Read the model definition and answer for the solid it produces. Units are mm, in the model's axes. A direction names the side the tool comes from. Give positions to 0.01 mm unless a question says otherwise; leave off trailing zeros. Write each loop counter-clockwise with the first axis right and the second up, starting at its lowest first coordinate (ties: lowest second). Pieces come first, ordered by that corner, then holes.
```python
from build123d import *

# Parameters (mm, degrees)
F3_DEPTH = 38.1
F4_W     = 88.9
F4_H     = 88.9
F5_DEPTH = 19.05
F7_W     = 114.3
F7_H     = 254
F8_DEPTH = 38.1


with BuildPart() as f3:
    # F2 (on offset) → F3 (new body)
    with BuildSketch(Plane.YZ.offset(19.05)):
        Polygon((729.5686676615, 1263.65), (652.579009265, 1308.1), (-102.6528778619, 0), (-610.6528778619, 0), (-610.6528778619, -88.9), (729.5686676615, -88.9), (729.5686676615, 0), (602.5686676615, 0), (301.2843338307, 521.8397737194), align=None)
        Polygon((499.9157897996, 0), (0, 0), (249.9578948998, 432.9397737194), align=None, mode=Mode.SUBTRACT)
    extrude(amount=F3_DEPTH)

    # F4 (on Right) → F5 (join, through all)
    with BuildSketch(Plane.YZ):
        with Locations((685.1186676615, -44.45)):
            Rectangle(F4_W, F4_H)
        Polygon((-559.8528778619, 0), (-610.6528778619, 0), (-610.6528778619, -88.9), (-470.9528778619, -88.9), align=None)
        Polygon((0, -88.9), (0, 0), (-102.6528778619, 0), (-153.9793167929, -88.9), align=None)
    extrude(amount=F5_DEPTH)

    # F6: F3 across plane


with BuildPart() as f3_1:
    add(f3.part)
    add(f3.part.mirror(Plane.YZ))

    # F7 (on face) → F8 (join)
    with BuildSketch(Plane(origin=(0, 0, 0), x_dir=(-1, 0, 0), z_dir=(0, 0.8660254038, -0.5))):
        with Locations((0, 1332.1373353229)):
            Rectangle(F7_W, F7_H)
    extrude(amount=F8_DEPTH)


solid = f3_1.part
```
Item 1: Section C-C (z = 476.5) is taken. Write down the section's boundary in (x, y).
Result set:
outline: (-57.15, 172.45) - (-19.05, 172.45) - (-19.05, 327.46) - (-57.15, 327.46) - close; (19.05, 172.45) - (57.15, 172.45) - (57.15, 327.46) - (19.05, 327.46) - close
Item 2: Section D-D (y = 321) is taken. Write down the section's boundary in (x, z).
Result set:
outline: (-57.15, -88.9) - (-19.05, -88.9) - (-19.05, 0) - (-57.15, 0) - close; (-57.15, 309.89) - (-19.05, 309.89) - (-19.05, 487.69) - (-57.15, 487.69) - close; (-57.15, 555.99) - (-19.05, 555.99) - (-19.05, 733.79) - (-57.15, 733.79) - close; (19.05, -88.9) - (57.15, -88.9) - (57.15, 0) - (19.05, 0) - close; (19.05, 309.89) - (57.15, 309.89) - (57.15, 487.69) - (19.05, 487.69) - close; (19.05, 555.99) - (57.15, 555.99) - (57.15, 733.79) - (19.05, 733.79) - close
Item 3: Find the intervals of material crossed by line 1 along Z through (x, y) = (-42, 465.5); line 2 along Z through (x, y) = (-32.5, 199); line 3 along Z through (x, y) = (34.5, 283), in increasing order.
Result set:
line 1: z = -88.9 to 0, 59.61 to 237.41, 806.27 to 984.07
line 2: z = -88.9 to 0, 344.68 to 522.48
line 3: z = -88.9 to 0, 375.71 to 667.97
Item 4: Determine the mould class of faces 1 (the flat face through (-37.833, 373.187, 219.5)), 2 (the flat face through (-37.83, 280.25, 663.21)), 3 (the flat face through (-57.15, 294, 368)) for opening direction Z: pulls with the +Z half, pulls with the -Z half, needs draft (parallel to the pull), parting line crosses it, or undercut.
Result set:
face 1: undercut
face 2: pulls with the +Z half
face 3: needs draft
Item 5: Which of the six approach directions +Z, -Z, +X, -X, +Y, -Y give full straight-line access (tool end or side, diameter ignored) to faces 4 (the flat face through (19.05, -334, -44)), 5 (the flat face through (0, -51, 0)), 6 (the flat face through (0.267, 666.958, 1155.205)), 7 (the flat face through (0.8, 699.95, 1136.15)), 8 (the flat face through (38, 253, 0))?
Result set:
face 4: +Z
face 5: +Z, +Y, -Y
face 6: +Z, -Y
face 7: +X, -X, +Y
face 8: +X, -X
Item 6: Section B-B (x = -40.5) is taken. Write down the section's boundary in (y, z), and give its area (3 significant figures).
Result set:
outline: (-610.65, -88.9) - (729.57, -88.9) - (729.57, 0) - (602.57, 0) - (301.28, 521.84) - (602.57, 1043.68) - (635.56, 1024.63) - (762.56, 1244.6) - (652.58, 1308.1) - (-102.65, 0) - (-610.65, 0) - close; hole (0, 0) - (499.92, 0) - (249.96, 432.94) - close
area: 310,000 mm2
Item 7: Section A-A (y = -202.5) is taken. Write down the section's boundary in (x, z), and give its area (3 significant figures).
Result set:
outline: (-57.15, -88.9) - (-19.05, -88.9) - (-19.05, 0) - (-57.15, 0) - close; (19.05, -88.9) - (57.15, -88.9) - (57.15, 0) - (19.05, 0) - close
area: 6,770 mm2
Item 8: Each of these flat-tipped pins is pushed along its axis until it touches: pin 1 Ø19 at (x, z) = (4.5, -25.5) entering from +Y; pin 2 Ø1.5 at (x, z) = (30, 447) entering from +Y; pin 3 Ø11.5 at (x, y) = (-5.5, -34.5) entering from +Z. Where does it stop, or does it pass through?
Result set:
pin 1: stops at y = 729.57
pin 2: stops at y = 344.93
pin 3: stops at z = 0
